```python
from build123d import *

# Parameters (mm, degrees)
SKETCH1_R           = 24.13
SKETCH1_R_2         = 20.32
BOSS_EXTRUDE1_DEPTH = 12.7
SKETCH2_W           = 12.7
SKETCH2_H           = 12.7
BOSS_EXTRUDE2_DEPTH = 12.7
SKETCH4_W           = 2.54
SKETCH4_H           = 58.988343485
CUT_EXTRUDE2_DEPTH  = 46.144990941
BOSS_EXTRUDE3_REACH = 68.615
BOSS_EXTRUDE3_START = 17.78
SKETCH5_W           = 35.97948453
SKETCH5_H           = 12.7
SKETCH6_W           = 22.86
SKETCH6_H           = 50.8
BOSS_EXTRUDE4_DEPTH = 12.7
SKETCH7_R           = 3.429
SKETCH7_W           = 10.16
SKETCH7_H           = 11.43
CUT_EXTRUDE3_DEPTH  = 91.9627717


with BuildPart() as part:
    # Sketch1 → Boss-Extrude1 (new body)
    with BuildSketch(Plane(origin=(0, 0, 0), x_dir=(1, 0, 0), z_dir=(0, 1, 0))):
        with Locations(Location((0, 0, 0), (0, 0, 270))):
            Circle(SKETCH1_R)
        with Locations(Location((0, 0, 0), (0, 0, 270))):
            Circle(SKETCH1_R_2, mode=Mode.SUBTRACT)
    extrude(amount=BOSS_EXTRUDE1_DEPTH)

    # Sketch2 → Boss-Extrude2 (add)
    with BuildSketch(Plane(origin=(0, 0, 0), x_dir=(1, 0, 0), z_dir=(0, 1, 0))):
        with Locations((0, 29.62948453)):
            Rectangle(SKETCH2_W, SKETCH2_H)
    extrude(amount=BOSS_EXTRUDE2_DEPTH)

    # Sketch4 → Cut-Extrude2 (cut, through all)
    with BuildSketch(Plane(origin=(0, 0, 0), x_dir=(1, 0, 0), z_dir=(0, 1, 0))):
        with Locations((0, 30.925816426)):
            Rectangle(SKETCH4_W, SKETCH4_H)
    extrude(amount=CUT_EXTRUDE2_DEPTH, mode=Mode.SUBTRACT)

    # Sketch5 → Boss-Extrude3 (add, up to next)
    with BuildSketch(Plane(origin=(6.35, 0, 0), x_dir=(0, 0, -1), z_dir=(1, 0, 0)).offset(BOSS_EXTRUDE3_START), mode=Mode.PRIVATE) as boss_extrude3_sk1:
        with Locations((17.989742265, 6.35)):
            Rectangle(SKETCH5_W, SKETCH5_H)
    boss_extrude3_tool1 = extrude(boss_extrude3_sk1.sketch, amount=-BOSS_EXTRUDE3_REACH, mode=Mode.PRIVATE) - part.part
    add(boss_extrude3_tool1.solids().sort_by_distance((24.13, 6.35, -17.989742))[0])

    # Sketch6 → Boss-Extrude4 (add)
    with BuildSketch(Plane(origin=(0, 12.7, 0), x_dir=(1, 0, 0), z_dir=(0, 1, 0))):
        with Locations((12.7, 61.37948453)):
            Rectangle(SKETCH6_W, SKETCH6_H)
    extrude(amount=-BOSS_EXTRUDE4_DEPTH)

    # Sketch7 → Cut-Extrude3 (cut, through all)
    with BuildSketch(Plane(origin=(0, 0, 0), x_dir=(1, 0, 0), z_dir=(0, 1, 0))):
        with Locations(Location((10.795, 80.42948453, 0), (0, 0, 270))):
            Circle(SKETCH7_R)
        with Locations((36.195, 80.42948453)):
            Circle(SKETCH7_R)
        with Locations((36.195, 67.72948453)):
            Circle(SKETCH7_R)
        with Locations(Location((10.795, 67.72948453, 0), (0, 0, 270))):
            Circle(SKETCH7_R)
        with Locations(Location((10.795, 55.02948453, 0), (0, 0, 270))):
            Circle(SKETCH7_R)
        with Locations((36.195, 55.02948453)):
            Circle(SKETCH7_R)
        with Locations(Location((10.795, 42.32948453, 0), (0, 0, 270))):
            Circle(SKETCH7_R)
        with Locations((36.195, 42.32948453)):
            Circle(SKETCH7_R)
        with Locations((11.43, 28.99448453)):
            Rectangle(SKETCH7_W, SKETCH7_H)
    extrude(amount=CUT_EXTRUDE3_DEPTH, mode=Mode.SUBTRACT)


solid = part.part
```
Check sheet for the modelled part. Datum: model origin and axes. Units: mm. A direction names the side the tool comes from. Give positions to 0.01 mm unless a question says otherwise; leave off trailing zeros. Write each loop counter-clockwise with the first axis right and the second up, starting at its lowest first coordinate (ties: lowest second). Pieces come first, ordered by that corner, then holes. Notation, with made-up numbers: (36, 36.5) -> (78, 36.5) arc R15 cw to (78, 40.5) -> close; hole circle Ø4 at (71.25, 65). An arc over 180 degrees is marked (long way). Use CSV: the item, a comma, the result in double quotes. Start each with the question number.
Q1. Tool access check on faces 1 (the flat face through (16.51, 6, -29)), 2 (the flat face through (1.27, 6, -53)), 3 (the flat face through (-4, 6, -35.979)). Record the directions out of +Z, -Z, +X, -X, +Y, -Y that give a thin tool (end or side, any length) a straight path to the whole face; none if there is none.
Q2. Cross-section at A-A on z = -15. Enter the section's corners in (x, y), and give its area (3 significant figures).
Q3. Cross-section at B-B on z = -29.5. Enter the section's corners in (x, y), and give its area (3 significant figures).
Q4. Scan lines: line 1 along X through (y, z) = (1.5, -27.5); line 2 along X through (y, z) = (1.5, -61.5); line 3 along Z through (x, y) = (18, 4.75). Record each from-to range of solid material in increasing order.
Q5. Cross-section at D-D on x = 3. Enter the section's corners in (y, z).
Q6. Release check for a two-part mould opening along X. For faces 4 (the flat face through (11, 6, -23.279)), 5 (the flat face through (-6.35, 6, -30)), 6 (the flat face through (11, 6, -34.709)), 7 (the flat face through (13, 6, -86.779)) record: +X half, -X half, draft (parallel to the pull), parting line (faces both ways), or undercut.
Q7. Cross-section at C-C on y = 7.75. Enter the section's corners in (x, z) (3 decimals), and give its area (3 significant figures).
Q8. Depth check by flat-ended pin: P1, Ø4, axis at y = 5.5, z = -46.5, coming from the -X side; P2, Ø4, axis at y = 8.5, z = -28, coming from the -X side; P3, Ø6, axis at x = 10.8, z = -55.03, coming from the +Y side; P4, Ø1.5, axis at x = -19, y = 2, coming from the +Z side. Enter the tip coordinate at first touch or a pass-through.
Working result:
1,face 1,"+Y, -Y"
1,face 2,"-Z, +Y, -Y"
1,face 3,"-Z, -X, +Y, -Y"
2,outline,"(-18.9, 0) -> (-13.71, 0) -> (-13.71, 12.7) -> (-18.9, 12.7) -> close; (13.71, 0) -> (24.13, 0) -> (24.13, 12.7) -> (13.71, 12.7) -> close"
2,area,"198 mm^2"
3,outline,"(-6.35, 0) -> (-1.27, 0) -> (-1.27, 12.7) -> (-6.35, 12.7) -> close; (1.27, 0) -> (6.35, 0) -> (6.35, 12.7) -> (1.27, 12.7) -> close; (16.51, 0) -> (24.13, 0) -> (24.13, 12.7) -> (16.51, 12.7) -> close"
3,area,"226 mm^2"
4,line 1,"x = -6.35 to -1.27, 1.27 to 6.35, 16.51 to 24.13"
4,line 2,"x = 1.27 to 24.13"
4,line 3,"z = -86.78 to -9.43, 9.43 to 16.07"
5,outline,"(0, -86.78) -> (12.7, -86.78) -> (12.7, -20.1) -> (0, -20.1) -> close; (0, 20.1) -> (12.7, 20.1) -> (12.7, 23.94) -> (0, 23.94) -> close"
6,face 4,"undercut"
6,face 5,"-X half"
6,face 6,"undercut"
6,face 7,"draft"
7,outline,"(-6.35, -35.979) -> (-1.27, -35.979) -> (-1.27, -20.28) arc R20.32 cw (long way) to (1.27, -20.28) -> (1.27, -86.779) -> (24.13, -86.779) -> (24.13, 0) arc R24.13 ccw (long way) to (-6.35, -23.279) -> close; hole (6.35, -34.709) -> (16.51, -34.709) -> (16.51, -23.279) -> (6.35, -23.279) -> close; hole circle Ø6.858 at (10.795, -80.429); hole circle Ø6.858 at (10.795, -67.729); hole circle Ø6.858 at (10.795, -55.029); hole circle Ø6.858 at (10.795, -42.329)"
7,area,"1,880 mm^2"
8,P1,"stops at x = 1.27"
8,P2,"stops at x = -6.35"
8,P3,"passes through"
8,P4,"stops at z = 15.79"
